CAD build for the part. Positions are in the model's coordinates, mm. A direction names the side the tool comes from. Round coordinates to 2 decimals unless told otherwise and drop trailing zeros. Write each loop counter-clockwise with the first axis right and the second up, starting at its lowest first coordinate (ties: lowest second). Pieces come first, ordered by that corner, then holes. Notation, with made-up numbers: (-6, 42) -> (40, 42) arc R32 cw to (40, 79) -> close; hole circle Ø5 at (22.25, 62.25). An arc over 180 degrees is marked (long way). Put each result on its own line as item: value. Start each with the question number.
1. Drill centre lines: line 1 (Y direction, x = -21, z = 0.7); line 2 (X direction, y = 40, z = 2.7). Where is each one in solid material? Low to high. Write a range as from..to.
2. Flat gauge pins, fed straight in: P1, Ø3, axis at x = 23, z = 2.5, coming from the -Y side; P2, Ø3, axis at x = -23, z = 2, coming from the +Y side; P3, Ø2, axis at y = 100.5, z = 2, coming from the -X side. Where does each tip first touch, or does it go through?
3. 3-axis set-ups, long thin cutter, end or side, ignore diameter. For faces 4 (the flat face through (20, 103, 3)), 5 (the flat face through (-23, 10, 3)), 6 (the flat face through (23, 72, 3)), 7 (the flat face through (-23, 46, 3)), 8 (the flat face through (23, 10, 3)): which of +Z, -Z, +X, -X, +Y, -Y reach the whole face in a straight line?
4. Pull direction Y, two halves, no side cores. Call faces 1 (the flat face through (26, 50, 3)), 2 (the flat face through (23, 64, 3)), 3 (the flat face through (23, 90, 3)): pulls with the +Y half, pulls with the -Y half, needs draft (parallel to the pull), parting line crosses it, or undercut.
5. Saw through at A-A on y = 22. List the corners of the cut face in (x, z), and give its area (3 significant figures).
Autodesk Inventor part; units mm, degrees
ref_plane "YZ Plane" through (0, 0, 0) normal (1, 0, 0) x (0, 1, 0)
ref_plane "XZ Plane" through (0, 0, 0) normal (0, 1, 0) x (-1, 0, 0)
ref_plane "XY Plane" through (0, 0, 0) normal (0, 0, 1) x (1, 0, 0)
sketch "Sketch1" plane through (0, 0, 0) normal (0, 0, 1) x (1, 0, 0)
  line L0 (0, 0) -> (-20, 0)
  line L1 (-20, 0) -> (-20, 10)
  line L2 (-20, 10) -> (-26, 10)
  line L3 (-26, 10) -> (-26, 18)
  line L4 (-26, 18) -> (-20, 18)
  line L5 (-20, 18) -> (-20, 28)
  line L6 (-20, 28) -> (-26, 28)
  line L7 (-26, 28) -> (-26, 36)
  line L8 (-26, 36) -> (-20, 36)
  line L9 (-20, 36) -> (-20, 46)
  line L10 (-20, 46) -> (-26, 46)
  line L11 (-26, 46) -> (-26, 54)
  line L12 (-26, 54) -> (-20, 54)
  line L13 (-20, 54) -> (-20, 64)
  line L14 (-20, 64) -> (-26, 64)
  line L15 (-26, 64) -> (-26, 72)
  line L16 (-26, 72) -> (-20, 72)
  line L17 (-20, 72) -> (-20, 82)
  line L18 (-20, 82) -> (-26, 82)
  line L19 (-26, 82) -> (-26, 90)
  line L20 (-26, 90) -> (-20, 90)
  line L21 (-20, 90) -> (-20, 115.388)
  line L22 (-20, 115.388) -> (0, 115.388)
  line L23 (0, 115.388) -> (0, 0) construction
  line L24 (0, 0) -> (20, 0)
  line L25 (20, 0) -> (20, 10)
  line L26 (20, 10) -> (26, 10)
  line L27 (26, 10) -> (26, 18)
  line L28 (26, 18) -> (20, 18)
  line L29 (20, 18) -> (20, 28)
  line L30 (26, 28) -> (26, 36)
  line L31 (26, 36) -> (20, 36)
  line L32 (20, 36) -> (20, 46)
  line L33 (20, 46) -> (26, 46)
  line L34 (26, 46) -> (26, 54)
  line L35 (26, 54) -> (20, 54)
  line L36 (20, 54) -> (20, 64)
  line L37 (20, 64) -> (26, 64)
  line L38 (26, 64) -> (26, 72)
  line L39 (26, 72) -> (20, 72)
  line L40 (20, 72) -> (20, 82)
  line L41 (20, 82) -> (26, 82)
  line L42 (26, 82) -> (26, 90)
  line L43 (26, 90) -> (20, 90)
  line L44 (20, 90) -> (20, 115.388)
  line L45 (20, 115.388) -> (0, 115.388)
  line L46 (20, 28) -> (26, 28)
  point P0 (-23, 90)
  dimension "d18" = 20
  dimension "d20" = 6
  dimension "d21" = 8
  dimension "d22" = 10
  dimension "d23" = 6
  dimension "d24" = 8
  dimension "d25" = 115.388
  dimension "d33" = 8
  dimension "d34" = 8
  dimension "d35" = 8
  dimension "d36" = 10
  dimension "d37" = 10
  dimension "d38" = 10
  dimension "d39" = 20
  dimension "d42" = 90
extrude "Extrusion1" add sketch "Sketch1" along normal blind 6
properties part number "sort support wall 3"
Return value:
1. line 1: y = 10..18, 28..36, 46..54, 64..72, 82..90
1. line 2: x = -20..20
2. P1: stops at y = 10
2. P2: stops at y = 90
2. P3: stops at x = -20
3. face 4: +Z, -Z, +X, +Y
3. face 5: +Z, -Z, -X, -Y
3. face 6: +Z, -Z, +X
3. face 7: +Z, -Z, -X
3. face 8: +Z, -Z, +X, -Y
4. face 1: needs draft
4. face 2: undercut
4. face 3: pulls with the +Y half
5. outline: (-20, 0) -> (20, 0) -> (20, 6) -> (-20, 6) -> close
5. area: 240 mm^2
